from build123d import *

# Parameters (mm, degrees)
BOSS_EXTRU_1_DEPTH      = 130
ESQUISSE2_W             = 2
ESQUISSE2_H             = 130
BOSS_EXTRU_2_DEPTH      = 96
ESQUISSE3_W             = 79.24305049
ESQUISSE3_H             = 150.673405859
ENL_V_MAT_EXTRU_1_DEPTH = 200
SKETCH1_W               = 504.296840386
SKETCH1_H               = 634.364351256
CUT_EXTRUDE1_DEPTH      = 345.11586261
SKETCH2_W               = 74.041478535
SKETCH2_H               = 186.425865598
CUT_EXTRUDE3_DEPTH      = 293.644673853
SKETCH3_W               = 110
SKETCH3_H               = 59.24305049
CUT_EXTRUDE4_DEPTH      = 293.644673853


with BuildPart() as part:
    # Esquisse1 → Boss.-Extru.1 (new body)
    with BuildSketch(Plane.XY):
        with BuildLine():
            Line((-99.346696614, 52.867973953), (258.521314081, -47.095157526))
            Line((258.521314081, -47.095157526), (259.05937636, -45.168894568))
            Line((259.05937636, -45.168894568), (-98.808634335, 54.794236911))
            ThreePointArc((-98.808634335, 54.794236911), (-99.208409273, 54.877062462), (-99.615727753, 54.904842474))
            Line((-99.615727753, 54.904842474), (-260.478685919, 54.904842474))
            ThreePointArc((-260.478685919, 54.904842474), (-262.600006262, 54.026162817), (-263.478685919, 51.904842474))
            Line((-263.478685919, 51.904842474), (-263.478685919, -47.095157526))
            Line((-263.478685919, -47.095157526), (-261.478685919, -47.095157526))
            Line((-261.478685919, -47.095157526), (-261.478685919, 51.904842474))
            ThreePointArc((-261.478685919, 51.904842474), (-261.1857927, 52.611949255), (-260.478685919, 52.904842474))
            Line((-260.478685919, 52.904842474), (-99.615727753, 52.904842474))
            ThreePointArc((-99.615727753, 52.904842474), (-99.479954927, 52.89558247), (-99.346696614, 52.867973953))
        make_face()
    extrude(amount=BOSS_EXTRU_1_DEPTH)

    # Esquisse2 → Boss.-Extru.2 (add)
    with BuildSketch(Plane.XZ.offset(47.095157526)):
        with Locations((-262.478685919, 65)):
            Rectangle(ESQUISSE2_W, ESQUISSE2_H)
    extrude(amount=BOSS_EXTRU_2_DEPTH)

    # Esquisse3 → Enlèv. mat.-Extru.1 (cut)
    with BuildSketch(Plane.ZY.offset(263.478685919)):
        with Locations((65, -17.758454597)):
            Rectangle(ESQUISSE3_W, ESQUISSE3_H)
    extrude(amount=-ENL_V_MAT_EXTRU_1_DEPTH, mode=Mode.SUBTRACT)

    # Sketch1 → Cut-Extrude1 (cut, through all)
    with BuildSketch(Plane(origin=(7.046316972, 25.225814758, 0), x_dir=(0.9631314790964218, -0.2690311394124084, 0), z_dir=(0.2690311394124084, 0.9631314790964218, 0))):
        with Locations((-363.353604044, 147.785884009)):
            Rectangle(SKETCH1_W, SKETCH1_H)
    extrude(amount=-CUT_EXTRUDE1_DEPTH, mode=Mode.SUBTRACT)

    # Sketch2 → Cut-Extrude3 (cut, through all)
    with BuildSketch(Plane(origin=(7.046316972, 25.225814758, 0), x_dir=(0.9631314790964218, -0.2690311394124084, 0), z_dir=(0.2690311394124084, 0.9631314790964218, 0))):
        with Locations((-128.650675605, -53.320838207)):
            Rectangle(SKETCH2_W, SKETCH2_H)
    extrude(amount=-CUT_EXTRUDE3_DEPTH, mode=Mode.SUBTRACT)

    # Sketch3 → Cut-Extrude4 (cut, through all)
    with BuildSketch(Plane(origin=(7.046316972, 25.225814758, 0), x_dir=(0.9631314790964218, -0.2690311394124084, 0), z_dir=(0.2690311394124084, 0.9631314790964218, 0))):
        with Locations((-18.224688862, -65)):
            Rectangle(SKETCH3_W, SKETCH3_H)
    extrude(amount=-CUT_EXTRUDE4_DEPTH, mode=Mode.SUBTRACT)


solid = part.part
The model under review builds one solid part; all positions refer to its coordinate system, in mm. A direction names the side the tool comes from. Round coordinates to 2 decimals unless told otherwise and drop trailing zeros. Loops run counter-clockwise (first coordinate to the right, second up) from the corner with the lowest first, then second, coordinate; pieces in that order, holes last. Notation, with made-up numbers: M 11,44 L 16,44 A21 cw 16,64 Z; hole C -0.5,87 d10. An arc over 180 degrees is marked long. Answer as CSV lines item,"result".
1. Insertion check: pin 1 Ø12 at (y, z) = (15, 54.5) entering from -X; pin 2 Ø0.6 at (y, z) = (44, 30) entering from -X; pin 3 Ø3 at (x, z) = (173.5, 59.5) entering from +Y. Each pin has a flat end and moves straight along its axis. Give the tip position at first contact, or say it passes through.
Outcome:
pin 1,"stops at x = 41.93"
pin 2,"stops at x = -63.48"
pin 3,"stops at y = -20.85"
2. To check wall thickness, follow L1, parallel to Y at x = 149, z = 92; L2, parallel to Y at x = 127.5, z = 87.5. State the ranges of each line that lie inside material, in increasing order. Write a range as [from, to].
Outcome:
L1,"y = [-16.5, -14.43]"
L2,"y = [-10.5, -8.42]"
3. Draft analysis for pull direction Z (two halves, no side actions). For faces 1 (the face through (129.116, -8.872, 64.09)), 2 (the face through (88, 2, 0)), 3 (the face through (88, 2, 130)), 4 (the face through (-73, 46, 25.378)), state which applies: pulls with the +Z half, pulls with the -Z half, needs draft (parallel to the pull), parting line crosses it, or undercut.
Outcome:
face 1,"needs draft"
face 2,"pulls with the -Z half"
face 3,"pulls with the +Z half"
face 4,"undercut"
4. We need section C-C (z = 99.5). Give the boundary of the cut face in (x, y), plus the area to 3 significant figures.
Outcome:
outline,"M -63.48,42.85 L 258.52,-47.1 L 259.06,-45.17 L -63.48,44.93 Z"
area,"669 mm2"
5. For faces 5 (the face through (-73, 46, 104.622)), 6 (the face through (123.814, -9.467, 64.09)), list the 3-axis set-ups (+Z, -Z, +X, -X, +Y, -Y) from which the entire face can be reached by the end or side of a thin tool; tool diameter is ignored.
Outcome:
face 5,"-X, +Y, -Y"
face 6,"+Z, -Z, -X, -Y"
6. We need section A-A (y = 28). Give the boundary of the cut face in (x, z), plus the area to 3 significant figures.
Outcome:
outline,"M -10.32,0 L -2.89,0 L -2.89,35.38 L -10.32,35.38 Z; M -10.32,94.62 L -2.89,94.62 L -2.89,130 L -10.32,130 Z"
area,"526 mm2"
7. We need section D-D (x = 208). Give the boundary of the cut face in (y, z).
Outcome:
outline,"M -32.98,0 L -30.91,0 L -30.91,130 L -32.98,130 Z"
8. We need section B-B (x = -39). Give the boundary of the cut face in (y, z), plus the area to 3 significant figures.
Outcome:
outline,"M 36.01,0 L 38.09,0 L 38.09,35.38 L 36.01,35.38 Z; M 36.01,94.62 L 38.09,94.62 L 38.09,130 L 36.01,130 Z"
area,"147 mm2"
